```python
from build123d import *

# Parameters (mm, degrees)
SKETCH1_W               = 82.55
SKETCH1_H               = 63.5
BOSS_EXTRUDE1_DEPTH     = 1.524
SKETCH2_OUTSIDE_W       = 105.382
SKETCH2_OUTSIDE_H       = 86.332
SKETCH2_OUTSIDE_R       = 1.54305
SKETCH2_OUTSIDE_R_2     = 1.5875
CUT_EXTRUDE1_DEPTH      = 53.096167815
SKETCH3_W               = 8.89
SKETCH3_H               = 1.524
BOSS_EXTRUDE2_DEPTH     = 22.86
CONVERT_SOLID2_START    = -28.6385
CONVERT_SOLID2_DEPTH    = 59.69
CONVERT_SOLID2_2_DEPTH  = 8.89
CONVERT_SOLID2_START_2  = 22.1615
CONVERT_SOLID2_3_DEPTH  = 8.89
CUT_EXTRUDE2_DEPTH      = 79.353236417
CUT_EXTRUDE2_DEPTH_BACK = 79.353236417
SKETCH12_R              = 1.5875


# Read off the part's stored shape, not the designer's step: Convert-Solid2
with BuildPart() as part:
    # Sketch1 → Boss-Extrude1 (new body)
    with BuildSketch(Plane.XY):
        Rectangle(SKETCH1_W, SKETCH1_H)
    extrude(amount=BOSS_EXTRUDE1_DEPTH)

    # Sketch2 outside → Cut-Extrude1 (cut, through all)
    # profile 1 of 9: a face of its own
    with BuildSketch(Plane.XY.offset(1.524)):
        Rectangle(SKETCH2_OUTSIDE_W, SKETCH2_OUTSIDE_H)
        with BuildLine():
            Line((-41.275, 8.347887239), (-41.275, -8.347887239))
            ThreePointArc((-41.275, -8.347887239), (-39.737239271, -14.405478713), (-35.496352053, -18.996121166))
            Line((-35.496352053, -18.996121166), (-19.031563189, -29.698233927))
            ThreePointArc((-19.031563189, -29.698233927), (-15.719742209, -31.22625909), (-12.110211137, -31.75))
            Line((-12.110211137, -31.75), (22.321500982, -31.75))
            ThreePointArc((22.321500982, -31.75), (27.931748365, -30.443644031), (32.387825644, -26.793326663))
            Line((32.387825644, -26.793326663), (38.641324662, -18.66377794))
            ThreePointArc((38.641324662, -18.66377794), (40.598566925, -15.009930266), (41.275, -10.920451277))
            Line((41.275, -10.920451277), (41.275, 10.920451277))
            ThreePointArc((41.275, 10.920451277), (40.598566925, 15.009930266), (38.641324662, 18.66377794))
            Line((38.641324662, 18.66377794), (31.0515, 28.53055))
            Line((31.0515, 28.53055), (31.0515, 31.75))
            Line((31.0515, 31.75), (22.1615, 31.75))
            Line((22.1615, 31.75), (22.1615, 28.702))
            Line((22.1615, 28.702), (-19.7485, 28.702))
            Line((-19.7485, 28.702), (-19.7485, 31.75))
            Line((-19.7485, 31.75), (-28.6385, 31.75))
            Line((-28.6385, 31.75), (-28.6385, 23.453725))
            Line((-28.6385, 23.453725), (-35.496352053, 18.996121166))
            ThreePointArc((-35.496352053, 18.996121166), (-39.737239271, 14.405478713), (-41.275, 8.347887239))
        make_face(mode=Mode.SUBTRACT)
    # profile 2 of 9: a face of its own
    with BuildSketch(Plane.XY.offset(1.524)):
        with Locations((-9.525, 22.225)):
            Circle(SKETCH2_OUTSIDE_R)
    # profile 3 of 9: a face of its own
    with BuildSketch(Plane.XY.offset(1.524)):
        with Locations((22.225, 22.225)):
            Circle(SKETCH2_OUTSIDE_R)
    # profile 4 of 9: a face of its own
    with BuildSketch(Plane.XY.offset(1.524)):
        with Locations((22.225, -22.225)):
            Circle(SKETCH2_OUTSIDE_R)
    # profile 5 of 9: a face of its own
    with BuildSketch(Plane.XY.offset(1.524)):
        with Locations((-9.525, -22.225)):
            Circle(SKETCH2_OUTSIDE_R)
    # profile 6 of 9: a face of its own
    with BuildSketch(Plane.XY.offset(1.524)):
        with Locations((34.925, -8.89)):
            Circle(SKETCH2_OUTSIDE_R_2)
    # profile 7 of 9: a face of its own
    with BuildSketch(Plane.XY.offset(1.524)):
        with Locations((34.925, 8.89)):
            Circle(SKETCH2_OUTSIDE_R_2)
    # profile 8 of 9: a face of its own
    with BuildSketch(Plane.XY.offset(1.524)):
        with Locations((-34.925, -8.89)):
            Circle(SKETCH2_OUTSIDE_R_2)
    # profile 9 of 9: a face of its own
    with BuildSketch(Plane.XY.offset(1.524)):
        with Locations((-34.925, 8.89)):
            Circle(SKETCH2_OUTSIDE_R_2)
    extrude(amount=-CUT_EXTRUDE1_DEPTH, mode=Mode.SUBTRACT)

    # Sketch3 → Boss-Extrude2 (add)
    with BuildSketch(Plane.XY.offset(1.524)):
        with Locations((-24.1935, 30.988)):
            Rectangle(SKETCH3_W, SKETCH3_H)
        with Locations((26.6065, 30.988)):
            Rectangle(SKETCH3_W, SKETCH3_H)
    extrude(amount=BOSS_EXTRUDE2_DEPTH)

    # Convert-Solid2 outline → Convert-Solid2 (cut)
    with BuildSketch(Plane.YZ.offset(CONVERT_SOLID2_START)):
        with BuildLine():
            ThreePointArc((31.75, 3.048), (30.857261469, 0.892738531), (28.702, 0))
            Line((28.702, 0), (31.75, 0))
            Line((31.75, 0), (31.75, 3.048))
        make_face()
    extrude(amount=CONVERT_SOLID2_DEPTH, mode=Mode.SUBTRACT)

    # Convert-Solid2 2 outline → Convert-Solid2 2 (add)
    with BuildSketch(Plane.YZ.offset(CONVERT_SOLID2_START)):
        with BuildLine():
            ThreePointArc((30.226, 3.048), (29.779630735, 1.970369265), (28.702, 1.524))
            Line((28.702, 1.524), (30.226, 1.524))
            Line((30.226, 1.524), (30.226, 3.048))
        make_face()
    extrude(amount=CONVERT_SOLID2_2_DEPTH)

    # Convert-Solid2 3 outline → Convert-Solid2 3 (add)
    with BuildSketch(Plane.YZ.offset(CONVERT_SOLID2_START_2)):
        with BuildLine():
            ThreePointArc((30.226, 3.048), (29.779630735, 1.970369265), (28.702, 1.524))
            Line((28.702, 1.524), (30.226, 1.524))
            Line((30.226, 1.524), (30.226, 3.048))
        make_face()
    extrude(amount=CONVERT_SOLID2_3_DEPTH)

    # Sketch12 → Cut-Extrude2 (cut, two sides: drawn at the far end of the back side and taken through both)
    with BuildSketch(Plane.XZ.offset(-30.226).offset(-CUT_EXTRUDE2_DEPTH_BACK)):
        with Locations(Location((-23.5585, 21.082, 0), (0, 0, 270))):
            Circle(SKETCH12_R)
        with Locations(Location((-23.5585, 11.0744, 0), (0, 0, 270))):
            Circle(SKETCH12_R)
        with Locations(Location((25.9715, 21.082, 0), (0, 0, 270))):
            Circle(SKETCH12_R)
        with Locations(Location((25.9715, 11.0744, 0), (0, 0, 270))):
            Circle(SKETCH12_R)
    extrude(amount=CUT_EXTRUDE2_DEPTH + CUT_EXTRUDE2_DEPTH_BACK, mode=Mode.SUBTRACT)


solid = part.part
```
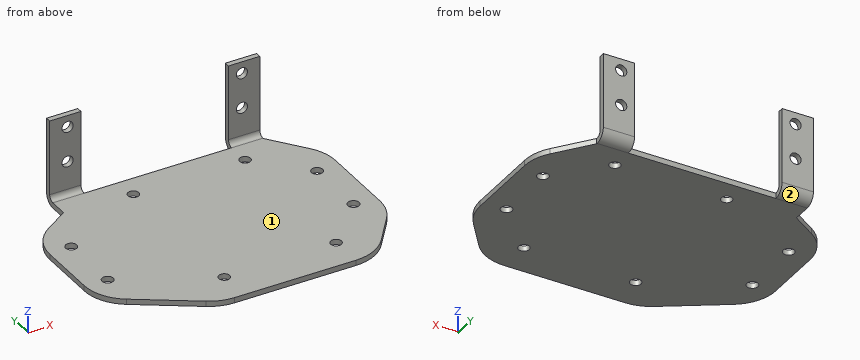
Check sheet for the modelled part. Datum: model origin and axes. Units: mm. Face numbers are marked on the shaded views. A direction names the side the tool comes from. Coordinates: 2 decimals unless noted, no trailing zeros. Order: outer loops, then holes, each group sorted by start corner. A loop starts at its lowest first (then second) coordinate and runs counter-clockwise, first axis right, second up. Notation, with made-up numbers: (0.5, 8.25) -> (47.5, 8.25) arc R24 ccw to (47.5, 44.25) -> close; hole circle Ø7 at (89.25, 43.25). An arc over 180 degrees is marked (long way). Write each question's results on one line, items separated by ' | '. Start each with the question number.
1) Depth check by flat-ended pin: pin 1 (5 mm diameter, centred on x = -34.925, y = 8.89, fed in from +Z); pin 2 (6.5 mm diameter, centred on y = 26, z = 18, fed in from -X); pin 3 (4.5 mm diameter, centred on x = -26, z = 17, fed in from -Y); pin 4 (2.5 mm diameter, centred on y = 30, z = 18, fed in from -X). Enter the tip coordinate at first touch or a pass-through.
2) Section check B-B (z = 16). Enter the section's corners in (x, y).
3) Set-up check for the marked faces 1 and 2: record each of +Z, -Z, +X, -X, +Y, -Y from which the full face is reachable in a straight line by a thin tool's end or side.
4) Section check A-A (z = 21.75). Enter the section's corners in (x, y), and give its area (3 significant figures).
5) Section check D-D (y = 5.5). Enter the section's corners in (x, z) (3 decimals).
6) Section check C-C (x = 16). Enter the section's corners in (y, z).
7) Material ranges on line 1 along Z through (x, y) = (-23, 16.5); line 2 along Y through (x, z) = (-25, 5.75), recorded low to high.
Checked values:
1) pin 1: z = 1.52 | pin 2: through | pin 3: y = 30.23 | pin 4: x = -28.64
2) outline: (-28.64, 30.23) -> (-19.75, 30.23) -> (-19.75, 31.75) -> (-28.64, 31.75) -> close; (22.16, 30.23) -> (31.05, 30.23) -> (31.05, 31.75) -> (22.16, 31.75) -> close
3) face 1: +Z, +X, -X, -Y | face 2: -Z, +X, -X, +Y
4) outline: (-28.64, 30.23) -> (-25, 30.23) -> (-25, 31.75) -> (-28.64, 31.75) -> close; (-22.12, 30.23) -> (-19.75, 30.23) -> (-19.75, 31.75) -> (-22.12, 31.75) -> close; (22.16, 30.23) -> (24.53, 30.23) -> (24.53, 31.75) -> (22.16, 31.75) -> close; (27.41, 30.23) -> (31.05, 30.23) -> (31.05, 31.75) -> (27.41, 31.75) -> close | area: 18.3 mm²
5) outline: (-41.275, 0) -> (41.275, 0) -> (41.275, 1.524) -> (-41.275, 1.524) -> close
6) outline: (-31.75, 0) -> (28.7, 0) -> (28.7, 1.52) -> (-31.75, 1.52) -> close
7) line 1: 0 to 1.52 | line 2: 30.23 to 31.75
